Verification items for the finished model (mm, model axes). Face numbers are marked on the shaded views. Round coordinates to 2 decimals unless told otherwise and drop trailing zeros. Order: outer loops, then holes, each group sorted by start corner. A loop starts at its lowest first (then second) coordinate and runs counter-clockwise, first axis right, second up. Notation, with made-up numbers: (-39, 21.5) -> (7, 21.5) arc R28 ccw to (7, 59.5) -> close; hole circle Ø9 at (-33.5, -29.5). An arc over 180 degrees is marked (long way). Put each result on its own line as item: value.
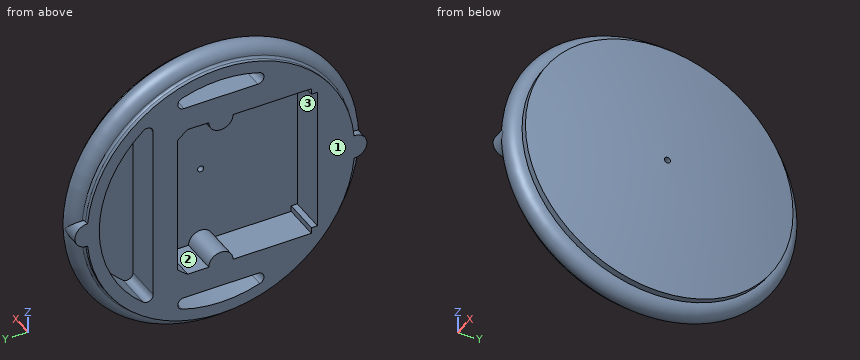
from build123d import *

# Parameters (mm, degrees)
BOSS_EXTRU_1_REACH = 6.224
ESQUISSE2_R        = 1
BOSS_EXTRU_2_DEPTH = 3.014801
BOSS_EXTRU_3_DEPTH = 1.4
CONG_3_R           = 0.5


with BuildPart() as part:
    # Esquisse1 → Révolution1 (revolve)
    with BuildSketch(Plane.XY):
        with BuildLine():
            Line((0, 10), (0, 11))
            Line((0, 11), (0.316784043, 11))
            ThreePointArc((0.316784043, 11), (0.445883488, 11.047247477), (0.513986703, 11.166666667))
            ThreePointArc((0.513986703, 11.166666667), (1.58362626, 11.996497189), (2.5, 11))
            Line((2.5, 11), (3, 11))
            ThreePointArc((3, 11), (3.90382078, 5.658215483), (4.224381403, 0.25))
            Line((4.224381403, 0.25), (3.014801263, 0.25))
            Line((3.014801263, 0.25), (3.014801263, 10))
            Line((3.014801263, 10), (0, 10))
        make_face()
    revolve(axis=Axis((-14.858593324, 0, 0), (1, 0, 0)))

    # Esquisse2 → Boss.-Extru.1 (add, up to next)
    with BuildSketch(Plane.ZY, mode=Mode.PRIVATE) as boss_extru_1_sk1:
        with Locations((0, 11)):
            Circle(ESQUISSE2_R)
    boss_extru_1_tool1 = extrude(boss_extru_1_sk1.sketch, amount=-BOSS_EXTRU_1_REACH, mode=Mode.PRIVATE) - part.part
    add(boss_extru_1_tool1.solids().sort_by_distance((0, 11, 0))[0])
    # Esquisse2 → Boss.-Extru.1 (add, up to next)
    with BuildSketch(Plane.ZY, mode=Mode.PRIVATE) as boss_extru_1_sk2:
        with Locations((0, -11)):
            Circle(ESQUISSE2_R)
    boss_extru_1_tool2 = extrude(boss_extru_1_sk2.sketch, amount=-BOSS_EXTRU_1_REACH, mode=Mode.PRIVATE) - part.part
    add(boss_extru_1_tool2.solids().sort_by_distance((0, -11, 0))[0])

    # Esquisse3 → Boss.-Extru.2 (add)
    with BuildSketch(Plane(origin=(0, 0, 0), x_dir=(0, 0, -1), z_dir=(1, 0, 0))):
        with BuildLine():
            Line((8.5, 0), (8.5, -5.267826876))
            ThreePointArc((8.5, -5.267826876), (0, -10), (-8.5, -5.267826876))
            Line((-8.5, -5.267826876), (-8.5, 0))
            Line((-8.5, 0), (-8.5, 5.267826876))
            ThreePointArc((-8.5, 5.267826876), (-8.407180778, 5.41473096), (-8.311822905, 5.56))
            Line((-8.311822905, 5.56), (8.311822905, 5.56))
            ThreePointArc((8.311822905, 5.56), (8.407180778, 5.41473096), (8.5, 5.267826876))
            Line((8.5, 5.267826876), (8.5, 0))
        make_face()
        with BuildLine():
            Line((6.5, -1), (6.5, -7.44))
            Line((6.5, -7.44), (6, -7.44))
            Line((6, -7.44), (6, -7.94))
            Line((6, -7.94), (-6, -7.94))
            Line((-6, -7.94), (-6, -7.44))
            Line((-6, -7.44), (-6.5, -7.44))
            Line((-6.5, -7.44), (-6.5, -1))
            ThreePointArc((-6.5, -1), (-5.5, 0), (-6.5, 1))
            Line((-6.5, 1), (-6.5, 3.56))
            Line((-6.5, 3.56), (6.5, 3.56))
            Line((6.5, 3.56), (6.5, 1))
            ThreePointArc((6.5, 1), (5.5, 0), (6.5, -1))
        make_face(mode=Mode.SUBTRACT)
    extrude(amount=BOSS_EXTRU_2_DEPTH)

    # Esquisse4 → Boss.-Extru.3 (add)
    with BuildSketch(Plane.ZY):
        with BuildLine():
            Line((-6.5, 3.56), (-5.809475019, 3.56))
            ThreePointArc((-5.809475019, 3.56), (-6.168925969, 3.153559893), (-6.5, 2.723689527))
            Line((-6.5, 2.723689527), (-6.5, 3.56))
        make_face()
        with BuildLine():
            Line((6.5, 3.56), (6.5, 2.723689527))
            ThreePointArc((6.5, 2.723689527), (6.168925969, 3.153559893), (5.809475019, 3.56))
            Line((5.809475019, 3.56), (6.5, 3.56))
        make_face()
    extrude(amount=-BOSS_EXTRU_3_DEPTH)

    # Congé3
    cong_3_edges = [part.edges().sort_by_distance(p)[0] for p in [
        (1.5074005, -5.267826876, -8.5),
        (1.5074005, -5.267826876, 8.5),
        (1.5074005, 5.267826876, 8.5),
        (1.5074005, 5.56, 8.311822905),
        (1.5074005, 5.56, -8.311822905),
        (1.5074005, 5.267826876, -8.5),
    ]]
    fillet(cong_3_edges, radius=CONG_3_R)


solid = part.part
Item 1: Gauge pin test, flat ends, axial feed: pin 1 Ø0.9 at (x, z) = (2, -1) entering from +Y; pin 2 Ø4 at (y, z) = (8, -9) entering from +X; pin 3 Ø0.8 at (y, z) = (3, -6) entering from +X. Record the tip position at first contact, or that the pin passes through.
Check sheet entries:
pin 1: stops at y = 11.97
pin 2: stops at x = 3.21
pin 3: stops at x = 3.83
Item 2: Section check A-A on x = 1.05. State how many separate pieces and enclosed holes the cut face has, then the cut area to 3 significant figures.
Check sheet entries:
separate pieces: 1
enclosed holes: 4
area: 230 mm^2
Item 3: Material ranges on L1, parallel to Y at x = 1.55, z = 4.5; L2, parallel to Z at x = 2.25, y = 6.5; L3, parallel to Y at x = 0.8, z = -7.25, recorded low to high. Write a range as [from, to].
Check sheet entries:
L1: y = [-11.12, -7.94], [3.56, 5.56], [8.93, 11.12]
L2: z = [-9.68, -7.6], [7.6, 9.68]
L3: y = [-9.2, 5.56], [6.89, 9.2]
Item 4: Section check B-B on x = 3.4. Record the boundary of the cut face in (y, z).
Check sheet entries:
outline: circle Ø18.09 at (0, 0); hole circle Ø0.5 at (0, 0)
Item 5: Release check for a two-part mould opening along X. For the marked faces 1, 2 and 3 record: +X half, -X half, draft (parallel to the pull), parting line (faces both ways), or undercut.
Check sheet entries:
face 1: -X half
face 2: undercut
face 3: draft
